Source: CAD feature listing. Evaluate the final solid. Frame: model axes, mm. Round coordinates to 2 decimals unless told otherwise and drop trailing zeros. Order: outer loops, then holes, each group sorted by start corner. A loop starts at its lowest first (then second) coordinate and runs counter-clockwise, first axis right, second up. Notation, with made-up numbers: (-5, 77) -> (32, 77) arc R32 ccw to (32, 105) -> close; hole circle Ø8 at (-13.5, -40). An arc over 180 degrees is marked (long way). Answer as CSV lines item,"result". Start each with the question number.
(1) Section query C-C (x = 58.5). Output: boundary loops of the cut face in (y, z).
(2) Section query A-A (x = -2.5). Output: boundary loops of the cut face in (y, z), plus the area to 3 significant figures.
(3) Section query B-B (y = 37.5). Output: boundary loops of the cut face in (x, z).
(4) Contact query for a flat-ended pin moving along its axis: P1, Ø7, axis at x = -27.5, y = 12.5, coming from the +Z side. Output: stop coordinate, or through.
(5) Line query: line 1 along Y through (x, z) = (-27.5, -1.15); line 2 along Y through (x, z) = (-2.5, 0.35). Output: solid intervals per line, ascending. Write a range as from..to.
```python
from build123d import *

# Parameters (mm, degrees)
SKETCH1_W           = 125
SKETCH1_H           = 100
SKETCH1_R           = 2.15
BOSS_EXTRUDE1_DEPTH = 2.5


with BuildPart() as part:
    # Sketch1 → Boss-Extrude1 (new, symmetric)
    with BuildSketch(Plane.XY):
        Rectangle(SKETCH1_W, SKETCH1_H)
        with Locations((-27.5, 37.5)):
            Circle(SKETCH1_R, mode=Mode.SUBTRACT)
        with Locations((-2.5, 37.5)):
            Circle(SKETCH1_R, mode=Mode.SUBTRACT)
        with Locations((-2.5, 12.5)):
            Circle(SKETCH1_R, mode=Mode.SUBTRACT)
        with Locations((-27.5, 12.5)):
            Circle(SKETCH1_R, mode=Mode.SUBTRACT)
        with Locations((-58.5, -46)):
            Circle(SKETCH1_R, mode=Mode.SUBTRACT)
        with Locations((58.5, -46)):
            Circle(SKETCH1_R, mode=Mode.SUBTRACT)
        with Locations((-29.25, -46)):
            Circle(SKETCH1_R, mode=Mode.SUBTRACT)
        with Locations((29.25, -46)):
            Circle(SKETCH1_R, mode=Mode.SUBTRACT)
    extrude(amount=BOSS_EXTRUDE1_DEPTH, both=True)


solid = part.part
```
Answer block:
1,outline,"(-50, -2.5) -> (-48.15, -2.5) -> (-48.15, 2.5) -> (-50, 2.5) -> close; (-43.85, -2.5) -> (50, -2.5) -> (50, 2.5) -> (-43.85, 2.5) -> close"
2,outline,"(-50, -2.5) -> (10.35, -2.5) -> (10.35, 2.5) -> (-50, 2.5) -> close; (14.65, -2.5) -> (35.35, -2.5) -> (35.35, 2.5) -> (14.65, 2.5) -> close; (39.65, -2.5) -> (50, -2.5) -> (50, 2.5) -> (39.65, 2.5) -> close"
2,area,"457 mm2"
3,outline,"(-62.5, -2.5) -> (-29.65, -2.5) -> (-29.65, 2.5) -> (-62.5, 2.5) -> close; (-25.35, -2.5) -> (-4.65, -2.5) -> (-4.65, 2.5) -> (-25.35, 2.5) -> close; (-0.35, -2.5) -> (62.5, -2.5) -> (62.5, 2.5) -> (-0.35, 2.5) -> close"
4,P1,"z = 2.5"
5,line 1,"-50..-47.25, -44.75..10.35, 14.65..35.35, 39.65..50"
5,line 2,"-50..10.35, 14.65..35.35, 39.65..50"
